from build123d import *

# Parameters (mm, degrees)
SKETCH_1_R          = 11
SKETCH_1_R_2        = 6.6
EXTRUDE_1_DEPTH     = 3
SKETCH_2_R          = 9.6
SKETCH_2_R_2        = 7.1
EXTRUDE_2_DEPTH     = 20
CHAMFER_1_SIZE      = 1
FILLET_1_R          = 1
SKETCH_3_R          = 11
SKETCH_3_R_2        = 9.6
EXTRUDE_3_DEPTH     = 1.5
SKETCH_4_R          = 7.1
SKETCH_4_R_2        = 6.6
EXTRUDE_4_DEPTH     = 8.5
SKETCH_5_R          = 7.5
CUT_EXTRUDE_1_DEPTH = 10
CHAMFER_2_SIZE      = 1


with BuildPart() as part:
    # 스케치1 → 보스-돌출1 (new body)
    with BuildSketch(Plane.XY):
        Circle(SKETCH_1_R)
        Circle(SKETCH_1_R_2, mode=Mode.SUBTRACT)
    extrude(amount=EXTRUDE_1_DEPTH)

    # 스케치2 → 보스-돌출2 (add)
    with BuildSketch(Plane.XY.offset(3)):
        Circle(SKETCH_2_R)
        Circle(SKETCH_2_R_2, mode=Mode.SUBTRACT)
    extrude(amount=EXTRUDE_2_DEPTH)

    # 모따기1
    chamfer_1_edges = [part.edges().sort_by_distance(p)[0] for p in [
        (-9.6, 0, 23),
    ]]
    chamfer(chamfer_1_edges, length=CHAMFER_1_SIZE)

    # 필렛1
    fillet_1_edges = [part.edges().sort_by_distance(p)[0] for p in [
        (-11, 0, 0),
    ]]
    fillet(fillet_1_edges, radius=FILLET_1_R)

    # 스케치3 → 보스-돌출3 (add)
    with BuildSketch(Plane.XY.offset(3)):
        Circle(SKETCH_3_R)
        Circle(SKETCH_3_R_2, mode=Mode.SUBTRACT)
    extrude(amount=EXTRUDE_3_DEPTH)

    # 스케치4 → 보스-돌출4 (add)
    with BuildSketch(Plane.XY.offset(3)):
        Circle(SKETCH_4_R)
        Circle(SKETCH_4_R_2, mode=Mode.SUBTRACT)
    extrude(amount=EXTRUDE_4_DEPTH)

    # 스케치5 → 컷-돌출1 (cut)
    with BuildSketch(Plane(origin=(0, 0, 0), x_dir=(-1, 0, 0), z_dir=(0, 0, -1))):
        Circle(SKETCH_5_R)
    extrude(amount=-CUT_EXTRUDE_1_DEPTH, mode=Mode.SUBTRACT)

    # 모따기2
    # the kernel refuses this chamfer: 1 mm, written as the material it adds along each edge
    with BuildSketch(Plane(origin=(0, 0, 10), x_dir=(-1, 0, 0), z_dir=(0, -1, 0))) as chamfer_2_piece_1_section:
        Polygon((7.5, CHAMFER_2_SIZE), (7.5 - CHAMFER_2_SIZE, 0), (7.5, 0), align=None)
    chamfer_2_piece_1 = revolve(axis=Axis((0, 0, 10), (0, 0, -1)), mode=Mode.PRIVATE)
    chamfer_2_piece_1 = chamfer_2_piece_1 - Plane(origin=(0, 0, 9.456358799), x_dir=(1, 0, 0), z_dir=(0, 0, -1)) * Cylinder(6.6, 30, mode=Mode.PRIVATE)
    add(chamfer_2_piece_1)
    # the kernel refuses this chamfer: 1 mm, written as the material it takes off along each edge
    with BuildSketch(Plane(origin=(0, 0, 0), x_dir=(-1, 0, 0), z_dir=(0, -1, 0))) as chamfer_2_2_piece_1:
        Polygon((7.5, -CHAMFER_2_SIZE), (7.5 + CHAMFER_2_SIZE, 0), (7.5, 0), align=None)
    revolve(axis=Axis((0, 0, 0), (0, 0, -1)), mode=Mode.SUBTRACT)


solid = part.part
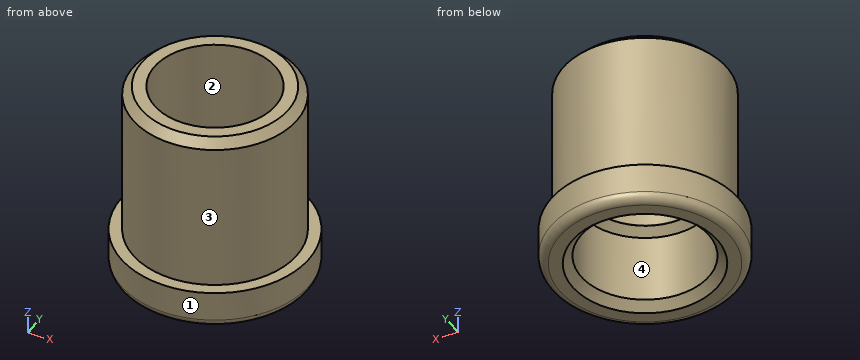
For this review, take the finished solid that the model builds, in its own axes (mm). Face numbers are marked on the shaded views. A direction names the side the tool comes from. Round coordinates to 2 decimals unless told otherwise and drop trailing zeros. Write each loop counter-clockwise with the first axis right and the second up, starting at its lowest first coordinate (ties: lowest second). Pieces come first, ordered by that corner, then holes. Notation, with made-up numbers: (32, 11.5) - (89, 11.5) arc R20 cw to (89, 38.5) - close; hole circle Ø3 at (54, -5). An arc over 180 degrees is marked (long way). Write item = value, one per line. Start each with the question number.
1. For the marked faces 1 and 2, list the 3-axis set-ups (+Z, -Z, +X, -X, +Y, -Y) from which the entire face can be reached by the end or side of a thin tool; tool diameter is ignored.
2. For pin 1 Ø5 at (x, z) = (8.5, 10) entering from +Y; pin 2 Ø8 at (x, y) = (0, 0) entering from -Z; pin 3 Ø10 at (x, z) = (-7.5, 5.5) entering from +Y; pin 4 Ø2 at (x, z) = (-5, 19.5) entering from +Y, all flat-tipped, find the tip position at first contact; note any pin that passes through.
3. Draft analysis for pull direction Y (two halves, no side actions). For the marked faces 3 and 4, state which applies: released by +Y, released by -Y, zero draft, split by the parting line, or undercut.
4. Consider section C-C on z = 10.5. State the section outline as (x, y) points.
5. Wall thickness on L1, parallel to Y at x = 0, z = 20.25; L2, parallel to Y at x = 0, z = 9.9; L3, parallel to X at y = 6.5, z = 20.5: over which ranges is each line inside the solid? List them lowest first.
6. Consider section D-D on z = 19.5. State the section outline as (x, y) points, plus the area to 3 significant figures.
7. Consider section A-A on y = 0. State the section outline as (x, z) points.
Evaluation:
q1.face_1 = +Z, -Z
q1.face_2 = +Z
q2.pin_1 = 7.49
q2.pin_2 = through
q2.pin_3 = 10.69
q2.pin_4 = 8.73
q3.face_3 = split by the parting line
q3.face_4 = undercut
q4.outline = circle Ø19.2 at (0, 0); hole circle Ø13.2 at (0, 0)
q5.L1 = -9.6 to -7.1, 7.1 to 9.6
q5.L2 = -9.6 to -6.6, 6.6 to 9.6
q5.L3 = -7.06 to -2.86, 2.86 to 7.06
q6.outline = circle Ø19.2 at (0, 0); hole circle Ø14.2 at (0, 0)
q6.area = 131 mm2
q7.outline = (-11, 1) arc R1 ccw to (-10, 0) - (-8.5, 0) - (-7.5, 1) - (-7.5, 9) - (-6.6, 9.9) - (-6.6, 11.5) - (-7.1, 11.5) - (-7.1, 23) - (-8.6, 23) - (-9.6, 22) - (-9.6, 4.5) - (-11, 4.5) - close; (6.6, 9.9) - (7.5, 9) - (7.5, 1) - (8.5, 0) - (10, 0) arc R1 ccw to (11, 1) - (11, 4.5) - (9.6, 4.5) - (9.6, 22) - (8.6, 23) - (7.1, 23) - (7.1, 11.5) - (6.6, 11.5) - close
